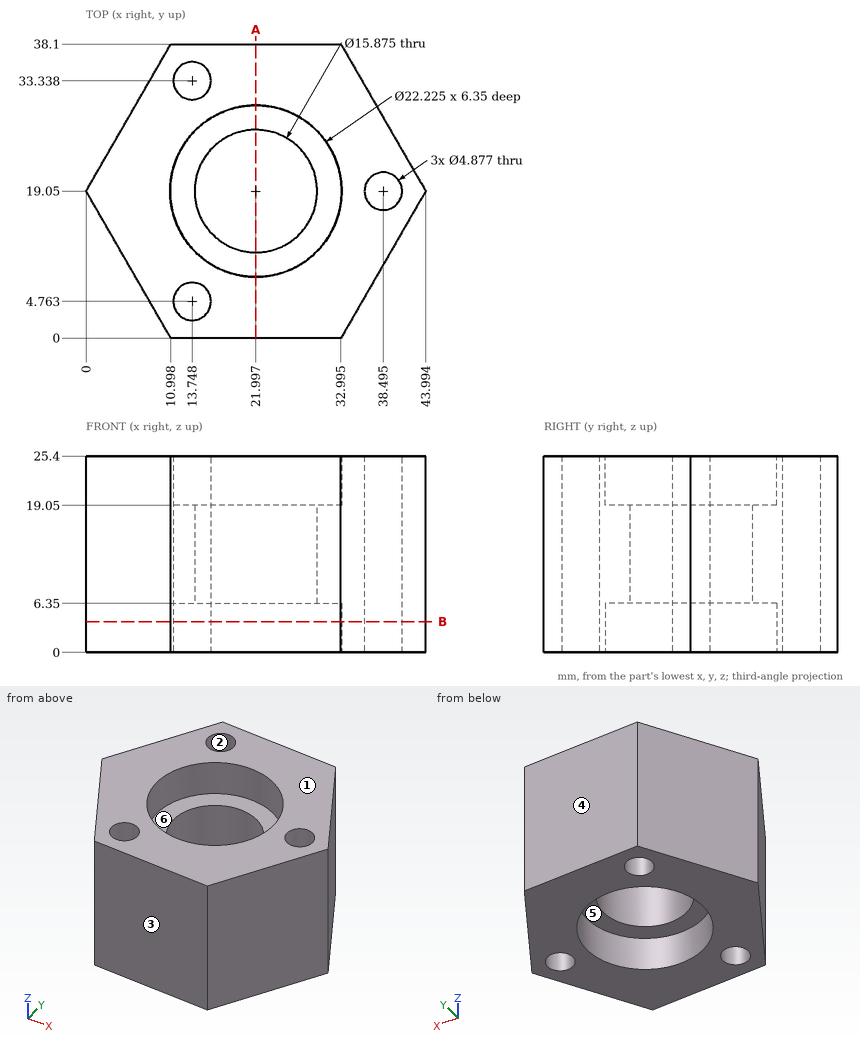
Here's the drawing with two shaded views (mm, measured from the low corner). I have some questions. A direction names the side the tool comes from. Round coordinates to 2 decimals unless told otherwise and drop trailing zeros. Order: outer loops, then holes, each group sorted by start corner. A loop starts at its lowest first (then second) coordinate and runs counter-clockwise, first axis right, second up. Notation, with made-up numbers: (16.5, 77) -> (37.5, 77) arc R19 cw to (37.5, 111) -> close; hole circle Ø11 at (-21, -21.5). An arc over 180 degrees is marked (long way). Return JSON: item names as keys, results as strings.
Q1. For pin 1 Ø5 at (x, y) = (28.5, 15.5) entering from -Z; pin 2 Ø1.5 at (y, z) = (4, 9) entering from +X; pin 3 Ø2 at (y, z) = (10, 7) entering from +X (1 decimal), each with a flat end and sliding along its axis, tell me the tip position at first contact or that it passes through.
Filled sheet:
{"pin 1": "stops at z = 6.35", "pin 2": "stops at x = 35.74", "pin 3": "stops at x = 39.3"}
Q2. If we mould it in two halves opening along Y, with no side actions, what happens to the marked faces 1, 2 and 3? For each: released by +Y, released by -Y, zero draft, split by the parting line, or undercut.
Filled sheet:
{"face 1": "zero draft", "face 2": "undercut", "face 3": "released by -Y"}
Q3. Which directions (+Z, -Z, +X, -X, +Y, -Y) give clear straight access to the entire face, cutting with the end or side of a thin tool? Please do the marked faces 4, 5 and 6.
Filled sheet:
{"face 4": "+Z, -Z, +X, -X, +Y", "face 5": "-Z", "face 6": "+Z"}
Q4. If we section it at A-A on x = 22: List the corners of the cut face in (y, z) for me, plus the area to 3 significant figures.
Filled sheet:
{"outline": "(0, 0) -> (7.94, 0) -> (7.94, 6.35) -> (11.11, 6.35) -> (11.11, 19.05) -> (7.94, 19.05) -> (7.94, 25.4) -> (0, 25.4) -> close; (26.99, 6.35) -> (30.16, 6.35) -> (30.16, 0) -> (38.1, 0) -> (38.1, 25.4) -> (30.16, 25.4) -> (30.16, 19.05) -> (26.99, 19.05) -> close", "area": "484 mm^2"}
Q5. If we section it at B-B on z = 4: Give the number of separate pieces and of enclosed holes in the cut face, plus the area to 3 significant figures.
Filled sheet:
{"separate pieces": "1", "enclosed holes": "4", "area": "813 mm^2"}
Q6. I need wall thicknesses on line 1 along X through (y, z) = (14.5, 23.25) (1 decimal); line 2 along Z through (x, y) = (31, 24.5); line 3 along Y through (x, z) = (23.5, 12) (1 decimal). Which ranges of each line are inside material? Lowest first, please. Write a range as from..to.
Filled sheet:
{"line 1": "x = 2.6..11.9, 32.1..41.4", "line 2": "z = 6.35..19.05", "line 3": "y = 0..11.3, 26.8..38.1"}
